Could you check a few things on this model? Use its own coordinates, in mm. A direction names the side the tool comes from. Round coordinates to 2 decimals unless told otherwise and drop trailing zeros. Loops run counter-clockwise (first coordinate to the right, second up) from the corner with the lowest first, then second, coordinate; pieces in that order, holes last. Notation, with made-up numbers: M 88,48 L 131,48 A16 ccw 131,56 Z; hole C 6.25,37.25 d11. An arc over 180 degrees is marked long. One line per item, written item: value. Start each with the question number.
Q1. Imagine slicing it at A-A (x = 35). Please give me the cut outline in (y, z).
Q2. Imagine slicing it at C-C (x = 106.5). Please give me the cut outline in (y, z), then the cut area to 3 significant figures.
Q3. Imagine slicing it at B-B (z = 2). Please give me the cut outline in (x, y), then the cut area to 3 significant figures.
Q4. I'm going to push flat-ended pins straight in: pin 1 Ø1 at (x, z) = (85, 19.5) entering from -Y; pin 2 Ø1.5 at (x, z) = (113.5, 8) entering from +Y; pin 3 Ø7 at (x, y) = (128, -7) entering from +Z. Where does each tip first touch, or does it pass through?
Q5. Please list where these lines run through material, in increasing order: line 1 along X through (y, z) = (-2.5, 20); line 2 along X through (y, z) = (2, 16.25); line 3 along Y through (x, z) = (85, 3).
Q6. Which directions (+Z, -Z, +X, -X, +Y, -Y) give clear straight access to the entire face, cutting with the end or side of a thin tool? Please do faces 4 (the face through (82.564, -1.38, 19.084)), 5 (the face through (114.37, -14.97, 6.34)).
Q7. Thinking about a two-plate mould opening in Y: for faces 1 (the face through (85, -2.8, 19)), 2 (the face through (69, 0, 0)), 3 (the face through (70.63, 0.55, 24.994)), which applies, released by +Y, released by -Y, zero draft, split by the parting line, or undercut?
Autodesk Inventor part; units mm, degrees
ref_plane "Plan de construction1" through (115, 25, 25) normal (0, 0, -1) x (-1, 0, 0)
ref_plane "Plan YZ" through (0, 0, 0) normal (1, 0, 0) x (0, 1, 0)
ref_plane "Plan XZ" through (0, 0, 0) normal (0, 1, 0) x (-1, 0, 0)
sketch "Esquisse1" plane through (0, 0, 0) normal (0, 0, 1) x (1, 0, 0)
  arc A0 (25, 25) -> (0, 0) centre (25, 0) ccw
  line L0 (25, 25) -> (115, 25)
  arc A1 (140, 0) -> (115, 25) centre (115, 0) ccw
  line L1 (0, 0) -> (140, 0)
  dimension "d0" = 90
  dimension "d1" = 25
revolve "Révolution1" add sketch "Esquisse1" angle 180 about axis through (0, 0, 0) along (1, 0, 0)
ref_plane "Plan de construction1" through (115, 25, 25) normal (0, 0, -1) x (-1, 0, 0)
sketch "Esquisse6" plane through (115, 25, 25) normal (0, 0, -1) x (-1, 0, 0)
  line L0 (76.7668, -25) -> (78.3834, -22.2)
  line L1 (78.3834, -22.2) -> (81.6166, -22.2)
  line L2 (81.6166, -22.2) -> (83.2332, -25)
  line L3 (83.2332, -25) -> (81.6166, -27.8)
  line L4 (81.6166, -27.8) -> (78.3834, -27.8)
  line L5 (78.3834, -27.8) -> (76.7668, -25)
  line L6 (90, 0) -> (90, -50)
  line L7 (26.7668, -25) -> (28.3834, -22.2)
  line L8 (28.3834, -22.2) -> (31.6166, -22.2)
  line L9 (31.6166, -22.2) -> (33.2332, -25)
  line L10 (33.2332, -25) -> (31.6166, -27.8)
  line L11 (31.6166, -27.8) -> (28.3834, -27.8)
  line L12 (28.3834, -27.8) -> (26.7668, -25)
  line L13 (30, -25) -> (26.7668, -25) construction
  line L14 (90, -25) -> (19.1163, -25) construction
  line L15 (80, -25) -> (76.7668, -25) construction
  point P0 (115, -25)
  dimension "d4" = 5.6
  dimension "d5" = 10
  dimension "d6" = 50
  dimension "d7" = 5.6
extrude "Extrusion1" cut sketch "Esquisse6" along normal blind 12
sketch "Esquisse7" plane through (115, 25, 25) normal (0, 0, -1) x (-1, 0, 0)
  circle A0 centre (80, -25) radius 3.2332 construction
  circle A1 centre (30, -25) radius 3.2332 construction
  circle A2 centre (80, -25) radius 1.7
  circle A3 centre (30, -25) radius 1.7
  point P0 (115, -25)
  point P1 (78.3834, -22.2)
  point P2 (28.3834, -22.2)
  point P3 (31.6166, -27.8)
  point P4 (28.3834, -27.8)
  point P5 (81.6166, -27.8)
  point P6 (78.3834, -27.8)
  dimension "d10" = 3.4
  dimension "d11" = 3.4
extrude "Extrusion2" cut sketch "Esquisse7" along normal blind 25
sketch "Esquisse8" plane through (115, 25, 25) normal (0, 0, -1) x (-1, 0, 0)
  line L0 (-0.0645, -24.9628) -> (-43.3013, 0) construction
  line L1 (-43.3013, 0) -> (-55.8013, -21.6506) construction
  line L2 (-55.8013, -21.6506) -> (9.1506, -59.1506) construction
  line L3 (9.1506, -59.1506) -> (21.6506, -37.5) construction
  line L4 (21.6506, -37.5) -> (-0.0645, -24.9628) construction
  arc A0 (0, 0) -> (0, -50) centre (0, -25) ccw
  line L5 (0, 0) -> (0, -50)
  line L6 (90, 0) -> (0, 0)
  line L7 (-13.9282, -33.1244) -> (-0.9378, -40.6244) construction
  circle A1 centre (-13.9282, -33.1244) radius 1.7
  circle A2 centre (-0.9378, -40.6244) radius 1.7
  point P0 (115, -25)
  dimension "d14" = 300
  dimension "d15" = 14
  dimension "d16" = 18
  dimension "d17" = 33
  dimension "d18" = 3.4
  dimension "d19" = 3.4
extrude "Extrusion3" cut sketch "Esquisse8" along normal blind 25 contours A2 L5 | L5 A2 | A1
sketch "Esquisse9" plane through (115, 25, 25) normal (0, 0, -1) x (-1, 0, 0)
  circle A0 centre (-13.9282, -33.1244) radius 3.25
  circle A1 centre (-0.9378, -40.6244) radius 3.25
  circle A2 centre (-13.9282, -33.1244) radius 1.7
  circle A3 centre (-0.9378, -40.6244) radius 1.7
  point P0 (115, -25)
  dimension "d22" = 6.5
  dimension "d23" = 6.5
extrude "Extrusion4" cut sketch "Esquisse9" along normal blind 12.5
equation "\"d7\" = d4"
equation "\"d11\" = d10"
equation "\"d19\" = d18"
equation "\"d23\" = d22"
properties part number "P1704_005_mainGaucheExterieur" material "PLA"
Report:
1. outline: M -25,0 L -1.7,0 L -1.7,13 L -2.8,13 L -2.8,24.84 A25 ccw Z; M 1.7,0 L 25,0 A25 ccw 2.8,24.84 L 2.8,13 L 1.7,13 Z
2. outline: M -25,0 L 25,0 A25 ccw Z
2. area: 982 mm²
3. outline: M 25,-24.92 L 115,-24.92 A24.92 ccw 115,24.92 L 25,24.92 A24.92 ccw Z; hole C 35,0 d3.4; hole C 85,0 d3.4; hole C 115.94,-15.62 d3.4; hole C 128.93,-8.12 d3.4
3. area: 6,400 mm²
4. pin 1: stops at y = -16.25
4. pin 2: stops at y = 23.93
4. pin 3: stops at z = 22.32
5. line 1: x = 10.21 to 33.21, 36.79 to 83.21, 86.79 to 129.79
5. line 2: x = 6.11 to 32.92, 37.08 to 82.92, 87.08 to 133.89
5. line 3: y = -24.82 to -1.7, 1.7 to 24.82
6. face 4: +Z
6. face 5: +Z, -Z
7. face 1: undercut
7. face 2: zero draft
7. face 3: split by the parting line
